The listing builds one solid part. Answer for the finished solid, in the listing's coordinates (mm). Give positions to 0.01 mm unless a question says otherwise; leave off trailing zeros. Loops run counter-clockwise (first coordinate to the right, second up) from the corner with the lowest first, then second, coordinate; pieces in that order, holes last. Notation, with made-up numbers: M 55,39 L 75,39 A25 cw 75,75 Z; hole C 78.25,-14 d4. An arc over 180 degrees is marked long. One line per item, written item: value. Start each with the question number.
Q1. Flat-ended cylindrical pins translate along their axes: pin 1 (4 mm diameter, centred on x = 258.5, z = 7, fed in from -Y); pin 2 (4.5 mm diameter, centred on y = 172.5, z = 5.5, fed in from +X). Find the tip coordinate at first contact, or state that the pin passes through.
Q2. A cutting plane is placed at D-D, the plane x = 299. Determine the outline of the cut face in (y, z).
Q3. A cutting plane is placed at B-B, the plane z = 2.25. Determine the outline of the cut face in (x, y), and give its area (3 significant figures).
Q4. A cutting plane is placed at A-A, the plane x = 437. Determine the outline of the cut face in (y, z).
Q5. A cutting plane is placed at C-C, the plane y = 498. Determine the outline of the cut face in (x, z).
Q6. Consider L1, parallel to Y at x = 404.5, z = 1.5; L2, parallel to X at y = 620.5, z = 4; L3, parallel to X at y = 181.5, z = 4.5. Determine where each line is inside the solid, lowest interval first.
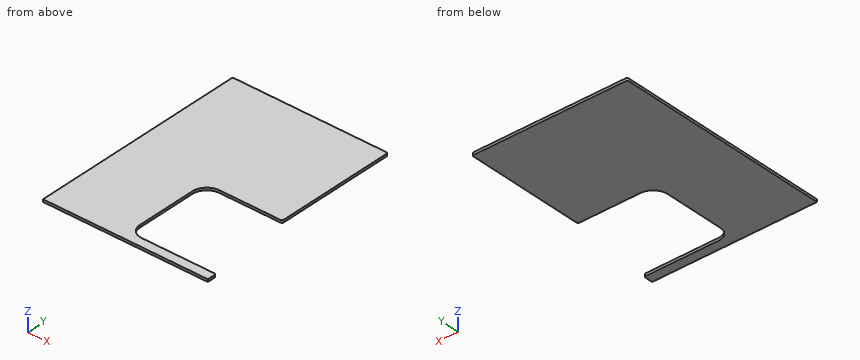
from build123d import *

# Parameters (mm, degrees)
BOSS_EXTRUDE1_DEPTH = 8.6


with BuildPart() as part:
    # Sketch1 → Boss-Extrude1 (new body)
    with BuildSketch(Plane.XY):
        with BuildLine():
            Line((0, 0), (0, 744.5))
            ThreePointArc((0, 744.5), (1.610912703, 748.389087297), (5.5, 750))
            Line((5.5, 750), (528.5, 750))
            ThreePointArc((528.5, 750), (532.389087297, 748.389087297), (534, 744.5))
            Line((534, 744.5), (534, 337.5))
            ThreePointArc((534, 337.5), (532.389087297, 333.610912703), (528.5, 332))
            Line((528.5, 332), (318.1, 332))
            ThreePointArc((318.1, 332), (282.744660941, 317.355339059), (268.1, 282))
            Line((268.1, 282), (268.1, 74.8))
            ThreePointArc((268.1, 74.8), (280.635829765, 44.535829765), (310.9, 32))
            Line((310.9, 32), (313, 32))
            Line((313, 32), (561.5, 32))
            ThreePointArc((561.5, 32), (565.389087297, 30.389087297), (567, 26.5))
            Line((567, 26.5), (567, 0))
            Line((567, 0), (0, 0))
        make_face()
    extrude(amount=BOSS_EXTRUDE1_DEPTH)


solid = part.part
Answer block:
1. pin 1: y = 0
1. pin 2: x = 268.1
2. outline: M 0,0 L 33.69,0 L 33.69,8.6 L 0,8.6 Z; M 328.21,0 L 750,0 L 750,8.6 L 328.21,8.6 Z
3. outline: M 0,0 L 567,0 L 567,26.5 A5.5 ccw 561.5,32 L 310.9,32 A42.8 cw 268.1,74.8 L 268.1,282 A50 cw 318.1,332 L 528.5,332 A5.5 ccw 534,337.5 L 534,744.5 A5.5 ccw 528.5,750 L 5.5,750 A5.5 ccw 0,744.5 Z
3. area: 323,000 mm^2
4. outline: M 0,0 L 32,0 L 32,8.6 L 0,8.6 Z; M 332,0 L 750,0 L 750,8.6 L 332,8.6 Z
5. outline: M 0,0 L 534,0 L 534,8.6 L 0,8.6 Z
6. L1: 0 to 32, 332 to 750
6. L2: 0 to 534
6. L3: 0 to 268.1
